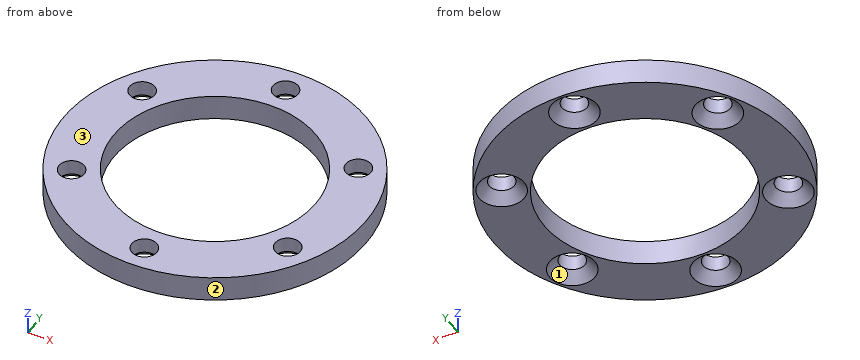
from build123d import *

# Parameters (mm, degrees)
SKETCH1_R           = 30
SKETCH1_R_2         = 20
SKETCH1_R_3         = 2.5
BOSS_EXTRUDE1_DEPTH = 5
CHAMFER1_SIZE       = 2


with BuildPart() as part:
    # Sketch1 → Boss-Extrude1 (new body)
    with BuildSketch(Plane.XY):
        Circle(SKETCH1_R)
        Circle(SKETCH1_R_2, mode=Mode.SUBTRACT)
        with Locations((0, 25)):
            Circle(SKETCH1_R_3, mode=Mode.SUBTRACT)
        with Locations((21.650635095, 12.5)):
            Circle(SKETCH1_R_3, mode=Mode.SUBTRACT)
        with Locations((21.650635095, -12.5)):
            Circle(SKETCH1_R_3, mode=Mode.SUBTRACT)
        with Locations((0, -25)):
            Circle(SKETCH1_R_3, mode=Mode.SUBTRACT)
        with Locations((-21.650635095, -12.5)):
            Circle(SKETCH1_R_3, mode=Mode.SUBTRACT)
        with Locations((-21.650635095, 12.5)):
            Circle(SKETCH1_R_3, mode=Mode.SUBTRACT)
    extrude(amount=BOSS_EXTRUDE1_DEPTH)

    # Chamfer1
    chamfer1_edges = [part.edges().sort_by_distance(p)[0] for p in [
        (19.150635095, -12.5, 0),
        (-2.5, -25, 0),
        (-24.150635095, -12.5, 0),
        (-24.150635095, 12.5, 0),
        (-2.5, 25, 0),
        (19.150635095, 12.5, 0),
    ]]
    chamfer(chamfer1_edges, length=CHAMFER1_SIZE)


solid = part.part
Input: part model. Units: mm. Frame: model coordinates. Face numbers are marked on the shaded views. Round coordinates to 2 decimals unless told otherwise and drop trailing zeros. Write each loop counter-clockwise with the first axis right and the second up, starting at its lowest first coordinate (ties: lowest second). Pieces come first, ordered by that corner, then holes.
1) Cut plane A-A (z = 4.25). Return the cut outline in (x, y), then the cut area to 3 significant figures.
2) Ray query, L1, parallel to Y at x = 0, z = 3.6; L2, parallel to Y at x = -22.5, z = 1.4; L3, parallel to Y at x = -2, z = 3.6. Return the intervals inside material, ascending.
3) Contact query for flat-ended pins moving along their axis: P1, Ø6.5, axis at x = 21.65, y = 12.5, coming from the +Z side; P2, Ø1, axis at y = -10, z = 3.5, coming from the -X side; P3, Ø3, axis at y = -22.5, z = 3.5, coming from the -X side. Output: stop coordinate, or through.
4) Draft query along X for the marked faces 1, 2 and 3. Return one class per face: pulls with the +X half, pulls with the -X half, needs draft (parallel to the pull), parting line crosses it, or undercut.
5) Cut plane D-D (y = 25). Return the cut outline in (x, z).
6) Cut plane C-C (y = -12.5). Return the cut outline in (x, z), then the cut area to 3 significant figures.
7) Cut plane B-B (x = 14.5). Return the cut outline in (y, z), then the cut area to 3 significant figures.
Geometry says:
1. outline: circle Ø60 at (0, 0); hole circle Ø5 at (-21.65, -12.5); hole circle Ø5 at (-21.65, 12.5); hole circle Ø40 at (0, 0); hole circle Ø5 at (0, -25); hole circle Ø5 at (0, 25); hole circle Ø5 at (21.65, -12.5); hole circle Ø5 at (21.65, 12.5)
1. area: 1,450 mm2
2. L1: y = -30 to -27.5, -22.5 to -20, 20 to 22.5, 27.5 to 30
2. L2: y = -19.84 to -15.48, -9.52 to 9.52, 15.48 to 19.84
2. L3: y = -29.93 to -26.5, -23.5 to -19.9, 19.9 to 23.5, 26.5 to 29.93
3. P1: stops at z = 5
3. P2: stops at x = -28.46
3. P3: stops at x = -21.42
4. face 1: undercut
4. face 2: parting line crosses it
4. face 3: needs draft
5. outline: (-16.58, 0) - (-4.5, 0) - (-2.5, 2) - (-2.5, 5) - (-16.58, 5) - close; (2.5, 2) - (4.5, 0) - (16.58, 0) - (16.58, 5) - (2.5, 5) - close
6. outline: (-27.27, 0) - (-26.15, 0) - (-24.15, 2) - (-24.15, 5) - (-27.27, 5) - close; (-19.15, 2) - (-17.15, 0) - (-15.61, 0) - (-15.61, 5) - (-19.15, 5) - close; (15.61, 0) - (17.15, 0) - (19.15, 2) - (19.15, 5) - (15.61, 5) - close; (24.15, 2) - (26.15, 0) - (27.27, 0) - (27.27, 5) - (24.15, 5) - close
6. area: 58.6 mm2
7. outline: (-26.26, 0) - (-13.77, 0) - (-13.77, 5) - (-26.26, 5) - close; (13.77, 0) - (26.26, 0) - (26.26, 5) - (13.77, 5) - close
7. area: 125 mm2
